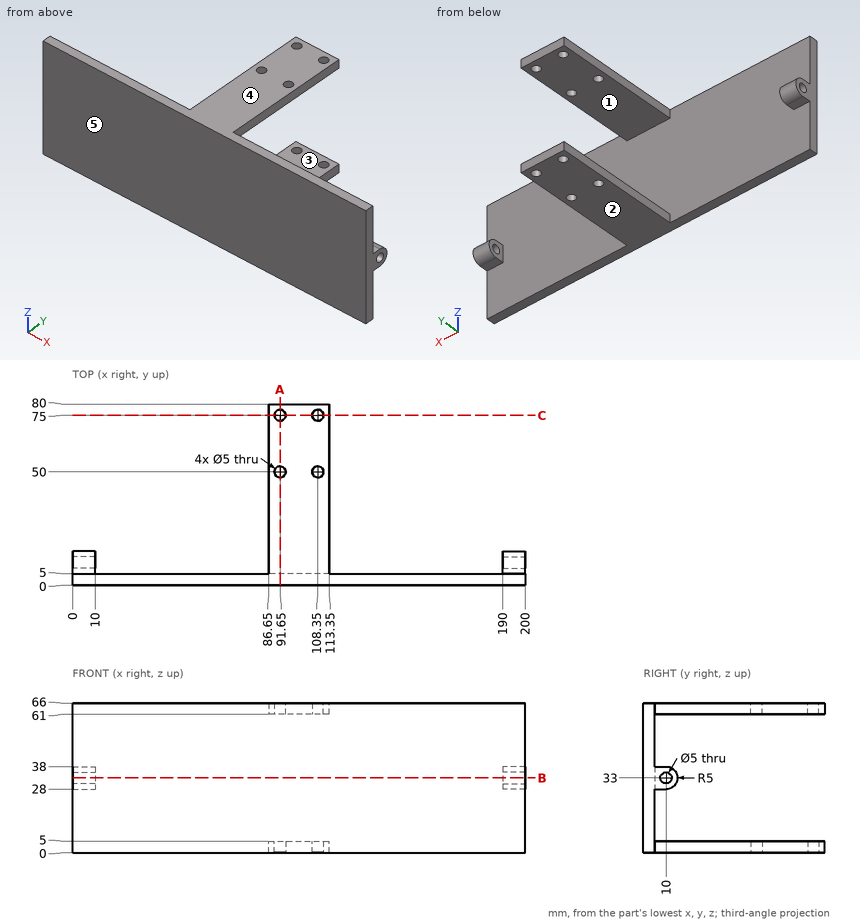
Input: dimensioned drawing with shaded views. Units: mm. Origin: part minimum x, y, z. A direction names the side the tool comes from. Coordinates: 2 decimals unless noted, no trailing zeros. Loops run counter-clockwise (first coordinate to the right, second up) from the corner with the lowest first, then second, coordinate; pieces in that order, holes last. Notation, with made-up numbers: M 46.25,35 L 85.25,35 A15 ccw 85.25,51 Z; hole C 44,12 d2. An arc over 180 degrees is marked long. One line per item, written item: value. Start each with the question number.
1) Cut plane C-C (y = 75). Return loops of the section in (x, z), then the cut area to 3 significant figures.
2) Pin query (flat end, axial travel): P1, Ø1.5, axis at x = 193, y = 8.5, coming from the +Z side; P2, Ø2.5, axis at x = 194.5, y = 8.5, coming from the -Z side; P3, Ø1.5, axis at x = 56, z = 35, coming from the +Y side. Return the tip coordinate at first contact, or that it passes through.
3) Material intervals for L1, parallel to X at y = 50, z = 3.2; L2, parallel to Y at x = 91.65, z = 64.25; L3, parallel to Z at x = 97, y = 71.5, sorted ascending. Write a range as from..to.
4) Cut plane A-A (x = 91.65). Return loops of the section in (y, z).
5) Cut plane B-B (z = 33). Return loops of the section in (x, y).
6) Draft query along Z for the marked faces 3, 4 and 5. Return one class per face: released by +Z, released by -Z, zero draft, split by the parting line, or undercut.
7) Reachability of the marked faces 1 and 2 from +Z, -Z, +X, -X, +Y, -Y: full face, straight path, thin tool, end or side. Return the list, or none.
Evaluation:
1. outline: M 86.65,0 L 89.15,0 L 89.15,5 L 86.65,5 Z; M 86.65,61 L 89.15,61 L 89.15,66 L 86.65,66 Z; M 94.15,0 L 105.85,0 L 105.85,5 L 94.15,5 Z; M 94.15,61 L 105.85,61 L 105.85,66 L 94.15,66 Z; M 110.85,0 L 113.35,0 L 113.35,5 L 110.85,5 Z; M 110.85,61 L 113.35,61 L 113.35,66 L 110.85,66 Z
1. area: 167 mm^2
2. P1: z = 38
2. P2: z = 28
2. P3: y = 5
3. L1: 86.65..89.15, 94.15..105.85, 110.85..113.35
3. L2: 0..47.5, 52.5..72.5, 77.5..80
3. L3: 0..5, 61..66
4. outline: M 0,0 L 47.5,0 L 47.5,5 L 5,5 L 5,61 L 47.5,61 L 47.5,66 L 0,66 Z; M 52.5,0 L 72.5,0 L 72.5,5 L 52.5,5 Z; M 52.5,61 L 72.5,61 L 72.5,66 L 52.5,66 Z; M 77.5,0 L 80,0 L 80,5 L 77.5,5 Z; M 77.5,61 L 80,61 L 80,66 L 77.5,66 Z
5. outline: M 0,0 L 200,0 L 200,7.5 L 190,7.5 L 190,5 L 10,5 L 10,7.5 L 0,7.5 Z; M 0,12.5 L 10,12.5 L 10,15 L 0,15 Z; M 190,12.5 L 200,12.5 L 200,15 L 190,15 Z
6. face 3: undercut
6. face 4: released by +Z
6. face 5: zero draft
7. face 1: +X, -X, +Y
7. face 2: -Z, +X, -X, +Y, -Y
